Autodesk Inventor part; units mm, degrees
ref_plane "YZ Plane" through (0, 0, 0) normal (1, 0, 0) x (0, 1, 0)
ref_plane "XZ Plane" through (0, 0, 0) normal (0, 1, 0) x (-1, 0, 0)
ref_plane "XY Plane" through (0, 0, 0) normal (0, 0, 1) x (1, 0, 0)
sketch "スケッチ1" plane through (0, 0, 0) normal (0, 1, 0) x (-1, 0, 0)
  arc A0 (0, -5) -> (-5, 0) centre (0, 0) ccw
  line L0 (0, -5) -> (-5, -5)
  line L1 (0, -5) -> (5, -5) construction
  line L2 (-5, -5) -> (-5, 0)
  dimension "d1" = 5
  dimension "d2" = 5
  dimension "d3" = 180
  dimension "d4" = 5
extrude "押し出し1" add sketch "スケッチ1" along normal blind 4.9
sketch "スケッチ2" plane through (0, 4.9, 0) normal (0, 1, 0) x (1, 0, 0)
  arc A0 (0, 5) -> (5, 0) centre (0, 0) ccw
  line L0 (0.0716, -4.9995) -> (0.0716, -6.9995)
  line L1 (0.0716, -6.9995) -> (3.5355, -3.5355)
  line L2 (0.0716, -6.9995) -> (4.9704, -6.9995) construction
  line L3 (0.0716, -4.9995) -> (3.5355, -3.5355)
  line L4 (4.3655, -2.4378) -> (6.0975, -3.4378)
  line L5 (6.0975, -3.4378) -> (4.8296, 1.2941)
  line L6 (4.3655, -2.4378) -> (4.8296, 1.2941)
  line L7 (4.2939, 2.5617) -> (6.0259, 3.5617)
  line L8 (6.0259, 3.5617) -> (1.2941, 4.8296)
  line L9 (4.2939, 2.5617) -> (1.2941, 4.8296)
  line L10 (-0.0716, 4.9995) -> (-0.0716, 6.9995)
  line L11 (-0.0716, 6.9995) -> (-3.5355, 3.5355)
  line L12 (-0.0716, 4.9995) -> (-3.5355, 3.5355)
  line L13 (-4.3655, 2.4378) -> (-6.0975, 3.4378)
  line L14 (-6.0975, 3.4378) -> (-4.8296, -1.2941)
  line L15 (-4.3655, 2.4378) -> (-4.8296, -1.2941)
  line L16 (-4.2939, -2.5617) -> (-6.0259, -3.5617)
  line L17 (-6.0259, -3.5617) -> (-1.2941, -4.8296)
  line L18 (-4.2939, -2.5617) -> (-1.2941, -4.8296)
  dimension "d7" = 2
  dimension "d8" = 45
  dimension "d41" = 360
sketch "スケッチ3" plane through (0, 4.9, 0) normal (0, 1, 0) x (1, 0, 0)
  point P0 (0, 0)
  point P1 (0, 0)
hole "穴1" at (0, 4.9, 0) direction (0, -1, 0) diameter 2 end through all
sketch "スケッチ4" plane through (5, 0, 0) normal (1, 0, 0) x (0, 0, -1)
  line L0 (0, 4.9) -> (5, 4.9)
  line L1 (5, 0) -> (5, 4.9)
  point P0 (0, 0)
  point P1 (2.5, 2.4)
  dimension "d28" = 2.5
  dimension "d29" = 2.5
hole "穴2" at (5, 2.4, -2.5) direction (-1, 0, 0) diameter 2.6 depth 5
sketch "スケッチ5" plane through (0, 4.9, 0) normal (0, 1, 0) x (1, 0, 0)
  point P0 (0, 0)
sketch "スケッチ7" plane through (0, 4.9, 0) normal (0, 1, 0) x (1, 0, 0)
  arc A0 (0, 5) -> (5, 0) centre (0, 0) ccw
  line L0 (0, 5) -> (-7, 5)
  line L1 (-7, 5) -> (-7, 4)
  line L2 (-7, 4) -> (-3, 4)
  line L3 (-3, 4) -> (0, 5)
  point P0 (-4.936, 0.7977)
  dimension "d35" = 7
  dimension "d36" = 1
extrude "押し出し4" add sketch "スケッチ7" against normal blind 4.9 contours A0 L2 L1 L0
extrude "押し出し5" add sketch "スケッチ2" against normal blind 4.9 contours A0 L17 L16
equation "\"d37\" = atumi"
properties part number "ikatire2b"
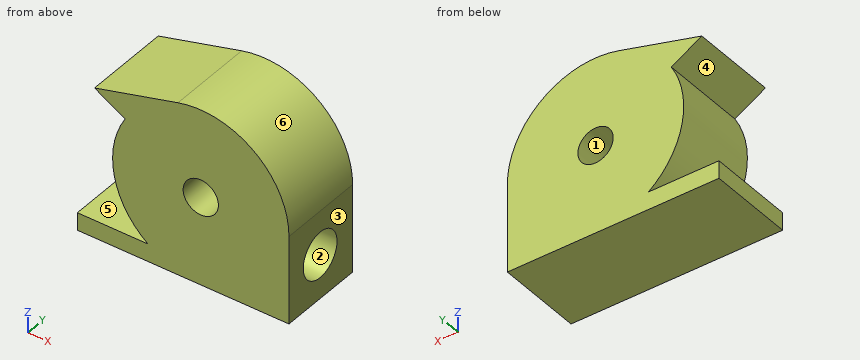
Verification items for the finished model (mm, model axes). Face numbers are marked on the shaded views. A direction names the side the tool comes from. Coordinates: 2 decimals unless noted, no trailing zeros. Order: outer loops, then holes, each group sorted by start corner. A loop starts at its lowest first (then second) coordinate and runs counter-clockwise, first axis right, second up.
1. Sectioned sample at A-A, the plane y = 1.25. Record the cut outline in (x, z), and give its area (3 significant figures).
Results found:
outline: (-7, -5) - (5, -5) - (5, -3.11) - (0, -3.11) - (0, -1.89) - (5, -1.89) - (5, 0) arc R5 ccw to (-1.29, 4.83) - (-6.03, 3.56) - (-4.29, 2.56) arc R5 ccw to (-3, -4) - (-7, -4) - close; hole circle Ø2 at (0, 0)
area: 82.2 mm2
2. Sectioned sample at B-B, the plane x = 3. Record the cut outline in (y, z), and give its area (3 significant figures).
Results found:
outline: (0, -5) - (4.9, -5) - (4.9, 4) - (0, 4) - close; hole circle Ø2.6 at (2.4, -2.5)
area: 38.8 mm2
3. Sectioned sample at C-C, the plane z = -2.25. Record the cut outline in (x, y).
Results found:
outline: (-4.47, 0) - (5, 0) - (5, 1.12) - (0, 1.12) - (0, 3.68) - (5, 3.68) - (5, 4.9) - (-4.47, 4.9) - close
4. Release check for a two-part mould opening along Z. For the marked faces 3, 4, 5 and 6 record: +Z half, -Z half, draft (parallel to the pull), parting line (faces both ways), or undercut.
Results found:
face 3: draft
face 4: undercut
face 5: undercut
face 6: +Z half
5. Go/stop test with flat-tipped pins: pin 1 Ø2 at (x, z) = (0.5, -2.5) entering from -Y; pin 2 Ø1 at (x, y) = (-1, 2.5) entering from +Z; pin 3 Ø1.3 at (y, z) = (2, -2.5) entering from +X; pin 4 Ø1.5 at (x, y) = (-2, 1) entering from +Z. Record where each tip stops, or that it passes through.
Results found:
pin 1: stops at y = 0
pin 2: stops at z = 4.97
pin 3: stops at x = 0
pin 4: stops at z = 4.84
6. Set-up check for the marked faces 1 and 2: record each of +Z, -Z, +X, -X, +Y, -Y from which the full face is reachable in a straight line by a thin tool's end or side.
Results found:
face 1: +Y, -Y
face 2: +X
7. Sectioned sample at D-D, the plane y = 2.2. Record the cut outline in (x, z), and give its area (3 significant figures).
Results found:
outline: (-7, -5) - (5, -5) - (5, -3.78) - (0, -3.78) - (0, -1.22) - (5, -1.22) - (5, 0) arc R5 ccw to (-1.29, 4.83) - (-6.03, 3.56) - (-4.29, 2.56) arc R5 ccw to (-3, -4) - (-7, -4) - close; hole circle Ø2 at (0, 0)
area: 75.4 mm2
8. Scan lines: line 1 (Y direction, x = 4.05, z = -2.5); line 2 (Z direction, x = 1.6, y = 2.4); line 3 (Z direction, x = 3.9, y = 2.4). Record each from-to range of solid material in increasing order.
Results found:
line 1: y = 0 to 1.1, 3.7 to 4.9
line 2: z = -5 to -3.8, -1.2 to 4.74
line 3: z = -5 to -3.8, -1.2 to 3.13
